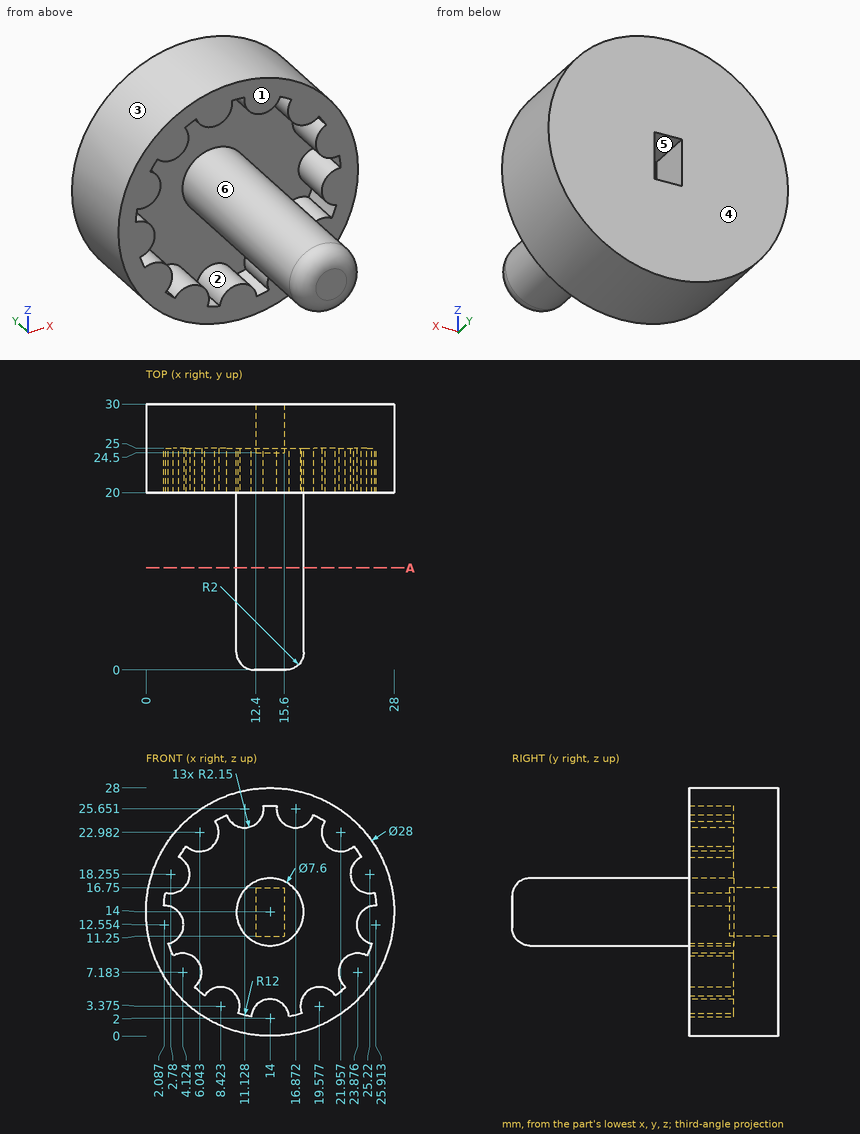
The drawing under review shows one solid part. Ordinate dimensions are in mm from its lowest x, y, z. A direction names the side the tool comes from. Give positions to 0.01 mm unless a question says otherwise; leave off trailing zeros. Loops run counter-clockwise (first coordinate to the right, second up) from the corner with the lowest first, then second, coordinate; pieces in that order, holes last. Notation, with made-up numbers: M 59.25,21 L 88.25,21 A31 ccw 88.25,46 Z; hole C 72.25,21 d10. An arc over 180 degrees is marked long. One line per question, with ' | ' between items. Start each with the question number.
1. To check wall thickness, follow L1, parallel to Z at x = 16.75, y = 20.5 (1 decimal); L2, parallel to Y at x = 15, z = 7; L3, parallel to Y at x = 3, z = 6.75. State the ranges of each line that lie inside material, in increasing order.
2. The part is to be moulded in two halves that separate along X. For the marked faces 1, 2 and 3, say which applies: released by +X, released by -X, zero draft, split by the parting line, or undercut.
3. Add section A-A (y = 11.5). Write out the cut boundary in (x, z).
4. For the marked faces 4, 5 and 6, list the 3-axis set-ups (+Z, -Z, +X, -X, +Y, -Y) from which the entire face can be reached by the end or side of a thin tool; tool diameter is ignored.
5. Insertion check: P1, Ø10, axis at y = 21.5, z = 5, coming from the -X side; P2, Ø2, axis at y = 6.5, z = 14.5, coming from the -X side; P3, Ø2, axis at x = 14, y = 4, coming from the +Z side. Each pin has a flat end and moves straight along its axis. Give the tip position at first contact, or say it passes through.
Worked out:
1) L1: z = 0.3 to 2.3, 11.4 to 16.6, 23.5 to 27.7 | L2: y = 25 to 30 | L3: y = 20 to 30
2) face 1: zero draft | face 2: undercut | face 3: split by the parting line
3) outline: C 14,14 d7.6
4) face 4: +Z, -Z, +X, -X, +Y | face 5: +Y | face 6: -Y
5) P1: stops at x = 0.58 | P2: stops at x = 10.2 | P3: stops at z = 17.8
